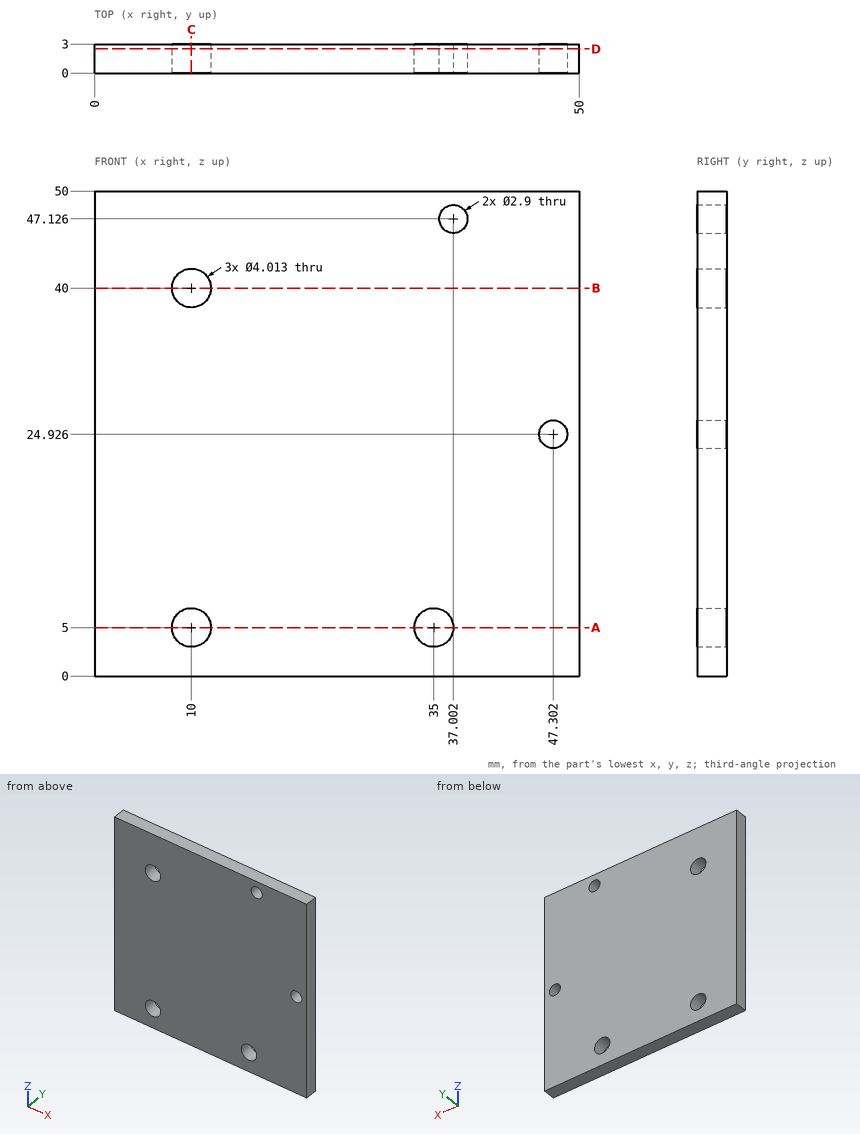
The drawing under review shows one solid part. Ordinate dimensions are in mm from its lowest x, y, z. Round coordinates to 2 decimals unless told otherwise and drop trailing zeros. Loops run counter-clockwise (first coordinate to the right, second up) from the corner with the lowest first, then second, coordinate; pieces in that order, holes last. Notation, with made-up numbers: (-24, -28) - (34, -28) arc R19 ccw to (34, 8) - close; hole circle Ø1 at (72.25, 19). An arc over 180 degrees is marked (long way). One line per item, written item: value. Start each with the question number.
1) Consider section C-C on x = 10. Give the boundary of the cut face in (y, z), then the cut area to 3 significant figures.
2) Consider section A-A on z = 5. Give the boundary of the cut face in (x, y), then the cut area to 3 significant figures.
3) To check wall thickness, follow L1, parallel to X at y = 0.9, z = 5; L2, parallel to Z at x = 10, y = 1.05; L3, parallel to X at y = 0.6, z = 6.5. State the ranges of each line that lie inside material, in increasing order. Write a range as from..to.
4) Consider section B-B on z = 40. Give the boundary of the cut face in (x, y).
5) Insertion check: pin 1 Ø5 at (x, z) = (10, 40) entering from +Y. The pin has a flat end and moves straight along its axis. Give the tip position at first contact, or say it passes through.
6) Consider section D-D on y = 2.5. Give the boundary of the cut face in (x, z), then the cut area to 3 significant figures.
Reported:
1. outline: (0, 0) - (3, 0) - (3, 2.99) - (0, 2.99) - close; (0, 7.01) - (3, 7.01) - (3, 37.99) - (0, 37.99) - close; (0, 42.01) - (3, 42.01) - (3, 50) - (0, 50) - close
1. area: 126 mm^2
2. outline: (0, 0) - (7.99, 0) - (7.99, 3) - (0, 3) - close; (12.01, 0) - (32.99, 0) - (32.99, 3) - (12.01, 3) - close; (37.01, 0) - (50, 0) - (50, 3) - (37.01, 3) - close
2. area: 126 mm^2
3. L1: x = 0..7.99, 12.01..32.99, 37.01..50
3. L2: z = 0..2.99, 7.01..37.99, 42.01..50
3. L3: x = 0..8.67, 11.33..33.67, 36.33..50
4. outline: (0, 0) - (7.99, 0) - (7.99, 3) - (0, 3) - close; (12.01, 0) - (50, 0) - (50, 3) - (12.01, 3) - close
5. pin 1: stops at y = 3
6. outline: (0, 0) - (50, 0) - (50, 50) - (0, 50) - close; hole circle Ø4.01 at (10, 5); hole circle Ø4.01 at (10, 40); hole circle Ø4.01 at (35, 5); hole circle Ø2.9 at (37, 47.13); hole circle Ø2.9 at (47.3, 24.93)
6. area: 2,450 mm^2
